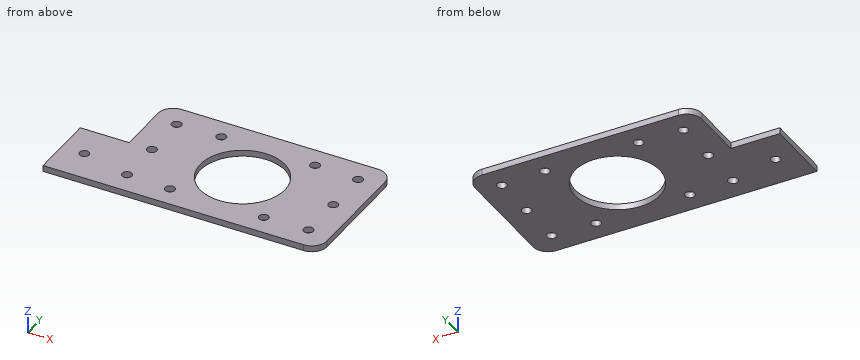
```python
from build123d import *

# Parameters (mm, degrees)
SKETCH1_W               = 75
SKETCH1_H               = 45
SKETCH1_R               = 14
SKETCH1_R_2             = 1.6
BOSS_EXTRUDE1_DEPTH     = 2.032
FILLET2_R               = 5
SKETCH2_R               = 1.6
CUT_EXTRUDE1_DEPTH      = 3.032
SKETCH4_W               = 21.18
SKETCH4_H               = 22.5
BOSS_EXTRUDE2_DEPTH     = 2.032
MOUNTING_HOLE_SKETCH_R  = 1.575
MOUNTING_HOLE_CUT_DEPTH = 3.032


with BuildPart() as part:
    # Sketch1 → Boss-Extrude1 (new body)
    with BuildSketch(Plane.XY):
        Rectangle(SKETCH1_W, SKETCH1_H)
        Circle(SKETCH1_R, mode=Mode.SUBTRACT)
        with Locations((-15.5, 15.5)):
            Circle(SKETCH1_R_2, mode=Mode.SUBTRACT)
        with Locations((15.5, 15.5)):
            Circle(SKETCH1_R_2, mode=Mode.SUBTRACT)
        with Locations((15.5, -15.5)):
            Circle(SKETCH1_R_2, mode=Mode.SUBTRACT)
        with Locations((-15.5, -15.5)):
            Circle(SKETCH1_R_2, mode=Mode.SUBTRACT)
    extrude(amount=BOSS_EXTRUDE1_DEPTH)

    # Fillet2
    fillet2_edges = [part.edges().sort_by_distance(p)[0] for p in [
        (37.5, -22.5, 1.016),
        (-37.5, -22.5, 1.016),
        (-37.5, 22.5, 1.016),
        (37.5, 22.5, 1.016),
    ]]
    fillet(fillet2_edges, radius=FILLET2_R)

    # Sketch2 → Cut-Extrude1 (cut, through all)
    with BuildSketch(Plane.XY.offset(2.032)):
        with Locations((-30, 0)):
            Circle(SKETCH2_R)
        with Locations((-30, 15)):
            Circle(SKETCH2_R)
        with Locations((-30, -15)):
            Circle(SKETCH2_R)
        with Locations((30, -15)):
            Circle(SKETCH2_R)
        with Locations((30, 15)):
            Circle(SKETCH2_R)
        with Locations((30, 0)):
            Circle(SKETCH2_R)
    extrude(amount=-CUT_EXTRUDE1_DEPTH, mode=Mode.SUBTRACT)

    # Sketch4 → Boss-Extrude2 (add)
    with BuildSketch(Plane(origin=(0, 0, 0), x_dir=(-1, 0, 0), z_dir=(0, 0, -1))):
        with Locations((43.09, -11.25)):
            Rectangle(SKETCH4_W, SKETCH4_H)
    extrude(amount=-BOSS_EXTRUDE2_DEPTH)

    # Mounting Hole Sketch → Mounting Hole Cut (cut, through all)
    with BuildSketch(Plane.XY.offset(2.032)):
        with Locations((-46.18, -11.25)):
            Circle(MOUNTING_HOLE_SKETCH_R)
    extrude(amount=-MOUNTING_HOLE_CUT_DEPTH, mode=Mode.SUBTRACT)


solid = part.part
```
Work out the finished part from the listing and answer in its coordinate system (mm). Round coordinates to 2 decimals unless told otherwise and drop trailing zeros. Loops run counter-clockwise (first coordinate to the right, second up) from the corner with the lowest first, then second, coordinate; pieces in that order, holes last. Notation, with made-up numbers: (-3, 51) -> (5, 51) arc R17 cw to (5, 69) -> close; hole circle Ø1 at (46.5, 89.5). An arc over 180 degrees is marked (long way). Write each question's results on one line, items separated by ' | '. Start each with the question number.
1. Section D-D (y = 9) is taken. Determine the outline of the cut face in (x, z), plus the area to 3 significant figures.
2. Section B-B (x = -46.18) is taken. Determine the outline of the cut face in (y, z) (3 decimals), plus the area to 3 significant figures.
3. Section A-A (x = -15.5) is taken. Determine the outline of the cut face in (y, z), plus the area to 3 significant figures.
4. Section C-C (z = 1.6) is taken. State how many separate pieces and enclosed holes the cut face has, plus the area to 3 significant figures.
5. Find the intervals of material crossed by probe 1 along Y at (x, z) = (30, 0.55); probe 2 along Y at (x, z) = (14.5, 0.25); probe 3 along X at (y, z) = (-12, 0.6), in increasing order. Write a range as from..to.
6. Given pin 1 Ø2.5 at (x, y) = (15.5, 15.5) entering from +Z; pin 2 Ø0.6 at (x, z) = (-49.5, 1) entering from +Y, each flat-ended and moving along its own axis, determine where each tip first touches the part or whether it passes through.
Evaluation:
1) outline: (-37.5, 0) -> (-10.72, 0) -> (-10.72, 2.03) -> (-37.5, 2.03) -> close; (10.72, 0) -> (37.5, 0) -> (37.5, 2.03) -> (10.72, 2.03) -> close | area: 109 mm2
2) outline: (-22.5, 0) -> (-12.825, 0) -> (-12.825, 2.032) -> (-22.5, 2.032) -> close; (-9.675, 0) -> (0, 0) -> (0, 2.032) -> (-9.675, 2.032) -> close | area: 39.3 mm2
3) outline: (-22.5, 0) -> (-17.1, 0) -> (-17.1, 2.03) -> (-22.5, 2.03) -> close; (-13.9, 0) -> (13.9, 0) -> (13.9, 2.03) -> (-13.9, 2.03) -> close; (17.1, 0) -> (22.5, 0) -> (22.5, 2.03) -> (17.1, 2.03) -> close | area: 78.4 mm2
4) separate pieces: 1 | enclosed holes: 12 | area: 3,020 mm2
5) probe 1: y = -22.5..-16.6, -13.4..-1.6, 1.6..13.4, 16.6..22.5 | probe 2: y = -22.5..-16.75, -14.25..14.25, 16.75..22.5 | probe 3: x = -53.68..-47.56, -44.8..-7.21, 7.21..37.5
6) pin 1: passes through | pin 2: stops at y = 0
